```python
from build123d import *

# Parameters (mm, degrees)
F0_R     = 12.6873
F0_R_2   = 7.6073
F0_R_3   = 5.55625
F1_DEPTH = 28.575
F2_R     = 7.6073
F3_DEPTH = 22.225
F4_R     = 5.55625
F5_DEPTH = 6.351


with BuildPart() as f1:
    # F0 (on Front) → F1 (new body)
    with BuildSketch(Plane.XZ):
        Circle(F0_R)
        Circle(F0_R_2, mode=Mode.SUBTRACT)
        Circle(F0_R_3)
        Circle(F0_R_2)
        Circle(F0_R_3, mode=Mode.SUBTRACT)
    extrude(amount=F1_DEPTH)

    # F2 (on face) → F3 (cut)
    with BuildSketch(Plane.XZ.offset(28.575)):
        Circle(F2_R)
    extrude(amount=-F3_DEPTH, mode=Mode.SUBTRACT)

    # F4 (on face) → F5 (cut, through all)
    with BuildSketch(Plane.XZ.offset(6.35)):
        Circle(F4_R)
    extrude(amount=-F5_DEPTH, mode=Mode.SUBTRACT)


solid = f1.part
```
Could you check a few things on this model? Use its own coordinates, in mm. A direction names the side the tool comes from. Round coordinates to 2 decimals unless told otherwise and drop trailing zeros. Loops run counter-clockwise (first coordinate to the right, second up) from the corner with the lowest first, then second, coordinate; pieces in that order, holes last.
Q1. I want a section at A-A (z = 0). Write out the boundary of the cut face in (x, y) (3 decimals).
Q2. Thinking about a two-plate mould opening in X: for faces 3 (the flat face through (5.5, -28.575, -5.5)), 4 (the cylindrical face through (5.3, -3.13, 1.67)), 5 (the cylindrical face through (-2.75, -14.087, -12.386)), which applies, pulls with the +X half, pulls with the -X half, needs draft (parallel to the pull), parting line crosses it, or undercut?
Q3. For P1, Ø13, axis at x = 0, z = 0, coming from the -Y side; P2, Ø4, axis at y = -11.5, z = -3.5, coming from the -X side; P3, Ø6, axis at y = -13.5, z = 6, coming from the +X side, each with a flat end and sliding along its axis, tell me the tip position at first contact or that it passes through.
Q4. On a 3-axis mill with a long thin cutter (end or side, diameter ignored), from which of +Z, -Z, +X, -X, +Y, -Y can I reach the whole of each face in a straight line? I mean faces 1 (the flat face through (5, 0, -3)), 2 (the cylindrical face through (7.256, -17.618, 2.285)). Say none if no direction works.
Q5. Please list where these lines run through material, in increasing order: L1, parallel to Z at x = 0, y = -23; L2, parallel to X at y = -5, z = 2.5; L3, parallel to X at y = -13, z = -3.5.
Q6. I want a section at D-D (y = -4.75). Write out the boundary of the cut face in (x, z).
Q7. I want a section at B-B (x = 0). Write out the boundary of the cut face in (y, z) (3 decimals).
Q8. I want a section at C-C (y = -14.5). Write out the boundary of the cut face in (x, z).
Answer below:
1. outline: (-12.687, -28.575) - (-7.607, -28.575) - (-7.607, -6.35) - (-5.556, -6.35) - (-5.556, 0) - (-12.687, 0) - close; (5.556, -6.35) - (7.607, -6.35) - (7.607, -28.575) - (12.687, -28.575) - (12.687, 0) - (5.556, 0) - close
2. face 3: needs draft
2. face 4: undercut
2. face 5: parting line crosses it
3. P1: stops at y = -6.35
3. P2: stops at x = -12.6
3. P3: stops at x = 12.33
4. face 1: +Z, -Z, +X, -X, +Y
4. face 2: -Y
5. L1: z = -12.69 to -7.61, 7.61 to 12.69
5. L2: x = -12.44 to -4.96, 4.96 to 12.44
5. L3: x = -12.19 to -6.75, 6.75 to 12.19
6. outline: circle Ø25.37 at (0, 0); hole circle Ø11.11 at (0, 0)
7. outline: (-28.575, -12.687) - (0, -12.687) - (0, -5.556) - (-6.35, -5.556) - (-6.35, -7.607) - (-28.575, -7.607) - close; (-28.575, 7.607) - (-6.35, 7.607) - (-6.35, 5.556) - (0, 5.556) - (0, 12.687) - (-28.575, 12.687) - close
8. outline: circle Ø25.37 at (0, 0); hole circle Ø15.21 at (0, 0)
